Could you check a few things on this drawing? It's one solid part, dimensions in mm from its lowest x, y, z. Coordinates: 2 decimals unless noted, no trailing zeros. Order: outer loops, then holes, each group sorted by start corner. A loop starts at its lowest first (then second) coordinate and runs counter-clockwise, first axis right, second up.
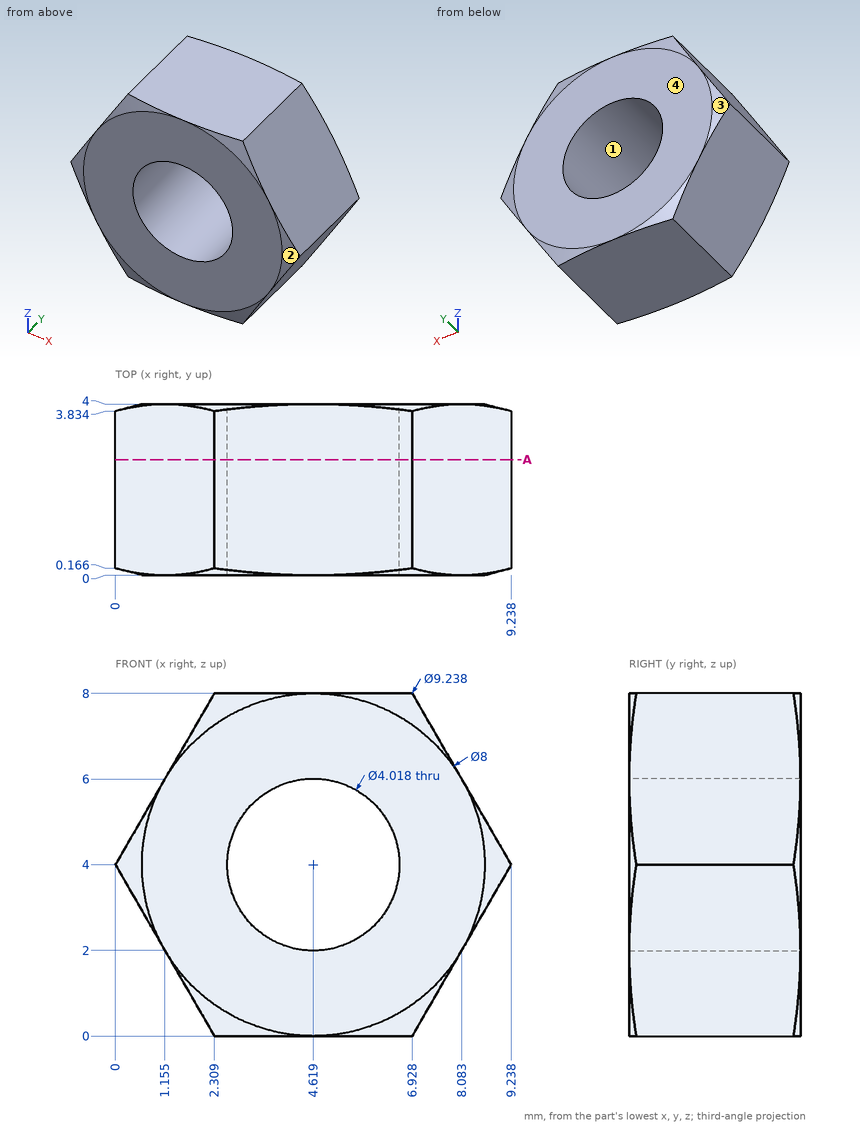
1. Thinking about a two-plate mould opening in X: for the marked faces 1, 2, 3 and 4, which applies, pulls with the +X half, pulls with the -X half, needs draft (parallel to the pull), parting line crosses it, or undercut?
Completed:
face 1: undercut
face 2: pulls with the +X half
face 3: pulls with the -X half
face 4: needs draft
2. Please list where these lines run through material, in increasing order: probe 1 along Z at (x, y) = (4, 3.6); probe 2 along Z at (x, y) = (5, 3.6); probe 3 along X at (y, z) = (1.15, 5.75) (1 decimal).
Completed:
probe 1: z = 0 to 2.09, 5.91 to 8
probe 2: z = 0 to 2.03, 5.97 to 8
probe 3: x = 1 to 3.6, 5.6 to 8.2
3. Imagine slicing it at A-A on y = 2.7. Please give me the cut outline in (x, z).
Completed:
outline: (0, 4) - (2.31, 0) - (6.93, 0) - (9.24, 4) - (6.93, 8) - (2.31, 8) - close; hole circle Ø4.02 at (4.62, 4)
4. I'm going to push a flat-ended pin straight in: pin 1 (1 mm diameter, centred on x = 4, z = 4.5, fed in from -Y). Where does the tip first touch, or does it pass through?
Completed:
pin 1: passes through
